Can you work these out from the model? Positions are in its coordinate system, mm. A direction names the side the tool comes from. Coordinates: 2 decimals unless noted, no trailing zeros. Write each loop counter-clockwise with the first axis right and the second up, starting at its lowest first coordinate (ties: lowest second). Pieces come first, ordered by that corner, then holes. Notation, with made-up numbers: (-38, -9.5) - (11, -9.5) arc R26 cw to (11, 26.5) - close; hole circle Ø3 at (83, 47). An arc over 180 degrees is marked (long way). Use one line per item in the form item = value. Start each with the question number.
(1) On a 3-axis mill with a long thin cutter (end or side, diameter ignored), from which of +Z, -Z, +X, -X, +Y, -Y can I reach the whole of each face in a straight line? I mean faces 1 (the face through (18.86, -6, 0)), 2 (the face through (-10.922, -6, 0)), 3 (the face through (38.1, -16, 0)), 4 (the face through (-18.86, -6, 0)). Say none if no direction works.
(2) If we section it at C-C on z = 0: Give the number of separate pieces and of enclosed holes in the cut face, then the cut area to 3 significant figures.
(3) If we section it at D-D on y = -14.5: Please give me the cut outline in (x, z) (3 decimals), then the cut area to 3 significant figures.
(4) Thinking about a two-plate mould opening in X: for faces 5 (the face through (-29, -12.7, 0)), 6 (the face through (-34.281, -15.831, 12.253)), 7 (the face through (-10.44, -12.25, 0.22)), 8 (the face through (10.922, -6, 0)), which applies, pulls with the +X half, pulls with the -X half, needs draft (parallel to the pull), parting line crosses it, or undercut?
(5) For pin 1 Ø3 at (x, z) = (3.5, -4) entering from +Y; pin 2 Ø1 at (y, z) = (-15, 9.5) entering from +X; pin 3 Ø5.5 at (y, z) = (-5.5, -4.5) entering from +X, each with a flat end and sliding along its axis, tell me the tip position at first contact or that it passes through.
(6) If we section it at A-A on y = -8.5: Please give me the cut outline in (x, z) (1 decimal).
(7) If I drill on probe 1 along Y at (x, z) = (16.75, 0); probe 2 along X at (y, z) = (4, 6); probe 3 along Y at (x, z) = (-3.5, 2), over which ranges is the centre line in solid material (lowest first)? Write a range as from..to.
```python
from build123d import *

# Parameters (mm, degrees)
BOSS_EXTRUDE1_DEPTH     = 15.875
CUT_EXTRUDE1_DEPTH      = 46.459081876
CUT_EXTRUDE1_DEPTH_BACK = 46.459081876
SKETCH2_R               = 4
FILLET1_R               = 12.7
FILLET2_R               = 1.5875
FILLET3_R               = 12.7


with BuildPart() as part:
    # Sketch1 → Boss-Extrude1 (new, symmetric)
    with BuildSketch(Plane.XY):
        Polygon((10.922, 7.9375), (18.8595, 7.9375), (18.8595, -12.7), (38.1, -12.7), (38.1, -19.05), (-38.1, -19.05), (-38.1, -12.7), (-18.8595, -12.7), (-18.8595, 7.9375), (-10.922, 7.9375), (-10.922, -12.7), (10.922, -12.7), align=None)
    extrude(amount=BOSS_EXTRUDE1_DEPTH, both=True)

    # Sketch2 → Cut-Extrude1 (cut, two sides: drawn at the far end of the back side and taken through both)
    with BuildSketch(Plane(origin=(0, 0, 0), x_dir=(0, 0, -1), z_dir=(1, 0, 0)).offset(-CUT_EXTRUDE1_DEPTH_BACK)):
        with Locations(Location((0, 0, 0), (0, 0, 90))):
            Circle(SKETCH2_R)
    extrude(amount=CUT_EXTRUDE1_DEPTH + CUT_EXTRUDE1_DEPTH_BACK, mode=Mode.SUBTRACT)

    # Fillet1
    fillet1_edges = [part.edges().sort_by_distance(p)[0] for p in [
        (14.89075, 7.9375, -15.875),
        (-14.89075, 7.9375, 15.875),
        (-14.89075, 7.9375, -15.875),
        (14.89075, 7.9375, 15.875),
    ]]
    fillet(fillet1_edges, radius=FILLET1_R)

    # Fillet2
    fillet2_edges = [part.edges().sort_by_distance(p)[0] for p in [
        (18.8595, -12.7, 0),
        (-18.8595, -12.7, 0),
        (-10.922, -12.7, 0),
        (10.922, -12.7, 0),
    ]]
    fillet(fillet2_edges, radius=FILLET2_R)

    # Fillet3
    fillet3_edges = [part.edges().sort_by_distance(p)[0] for p in [
        (38.1, -15.875, -15.875),
        (-38.1, -15.875, -15.875),
        (-38.1, -15.875, 15.875),
        (38.1, -15.875, 15.875),
    ]]
    fillet(fillet3_edges, radius=FILLET3_R)


solid = part.part
```
Reported:
q1.face_1 = +Z, -Z, +X, +Y
q1.face_2 = +Z, -Z, +Y
q1.face_3 = +Z, -Z, +X, +Y, -Y
q1.face_4 = +Z, -Z, -X, +Y
q2.separate_pieces = 3
q2.enclosed_holes = 0
q2.area = 687 mm2
q3.outline = (-38.1, -3.175) arc R12.7 ccw to (-25.4, -15.875) - (25.4, -15.875) arc R12.7 ccw to (38.1, -3.175) - (38.1, 3.175) arc R12.7 ccw to (25.4, 15.875) - (-25.4, 15.875) arc R12.7 ccw to (-38.1, 3.175) - close
q3.area = 2,280 mm2
q4.face_5 = needs draft
q4.face_6 = pulls with the -X half
q4.face_7 = undercut
q4.face_8 = undercut
q5.pin_1 = -12.7
q5.pin_2 = 36.69
q5.pin_3 = 18.86
q6.outline = (-18.9, -15.9) - (-10.9, -15.9) - (-10.9, 15.9) - (-18.9, 15.9) - close; (10.9, -15.9) - (18.9, -15.9) - (18.9, 15.9) - (10.9, 15.9) - close
q7.probe_1 = -19.05..-4, 4..7.94
q7.probe_2 = -18.86..-10.92, 10.92..18.86
q7.probe_3 = -19.05..-12.7
